from build123d import *

# Parameters (mm, degrees)
BOSS_EXTRUDE1_DEPTH = 25.4


with BuildPart() as part:
    # Sketch1 → Boss-Extrude1 (new body)
    with BuildSketch(Plane(origin=(0, 0, 0), x_dir=(1, 0, 0), z_dir=(0, 1, 0))):
        with BuildLine():
            Line((-2.032, 11.247927631), (-1.27, 14.803927631))
            Line((-1.27, 14.803927631), (1.27, 14.803927631))
            Line((1.27, 14.803927631), (2.032, 11.247927631))
            ThreePointArc((2.032, 11.247927631), (8.082230509, 8.082230509), (11.247927631, 2.032))
            Line((11.247927631, 2.032), (14.803927631, 1.27))
            Line((14.803927631, 1.27), (14.803927631, -1.27))
            Line((14.803927631, -1.27), (11.247927631, -2.032))
            ThreePointArc((11.247927631, -2.032), (8.082230509, -8.082230509), (2.032, -11.247927631))
            Line((2.032, -11.247927631), (1.27, -14.803927631))
            Line((1.27, -14.803927631), (-1.27, -14.803927631))
            Line((-1.27, -14.803927631), (-2.032, -11.247927631))
            ThreePointArc((-2.032, -11.247927631), (-8.082230509, -8.082230509), (-11.247927631, -2.032))
            Line((-11.247927631, -2.032), (-14.803927631, -1.27))
            Line((-14.803927631, -1.27), (-14.803927631, 1.27))
            Line((-14.803927631, 1.27), (-11.247927631, 2.032))
            ThreePointArc((-11.247927631, 2.032), (-8.082230509, 8.082230509), (-2.032, 11.247927631))
        make_face()
        with BuildLine():
            Line((-2.032, -1.524), (2.032, -1.524))
            ThreePointArc((2.032, -1.524), (0, 2.54), (-2.032, -1.524))
        make_face(mode=Mode.SUBTRACT)
    extrude(amount=BOSS_EXTRUDE1_DEPTH)


solid = part.part
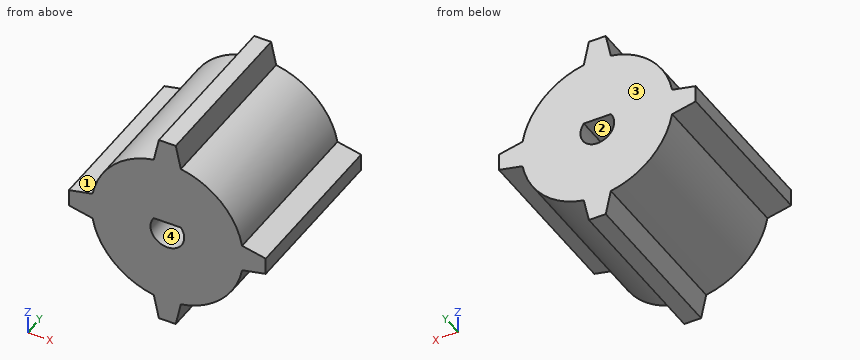
Model file for the job. Use its own axes, mm. Face numbers are marked on the shaded views. Round coordinates to 2 decimals unless told otherwise and drop trailing zeros. Order: outer loops, then holes, each group sorted by start corner. A loop starts at its lowest first (then second) coordinate and runs counter-clockwise, first axis right, second up. Notation, with made-up numbers: M 70,0.5 L 82,0.5 A28 cw 82,33.5 Z; hole C 49,-26.5 d11. An arc over 180 degrees is marked long. Write each question's results on one line, items separated by ' | '. Start each with the question number.
(1) Two-plate mould, pull along X, no slides. Class the marked faces 1, 2, 3 and 4: pulls with the +X half, pulls with the -X half, needs draft (parallel to the pull), parting line crosses it, or undercut.
(2) Saw through at B-B, the plane y = 13.75. Give the cut face in (x, z), then the cut area to 3 significant figures.
(3) Saw through at D-D, the plane x = 4.5. Give the cut face in (y, z), then the cut area to 3 significant figures.
(4) Probe probe 1 along X at (y, z) = (6, 0); probe 2 along X at (y, z) = (12.25, -2.25); probe 3 along Z at (x, y) = (-3.25, 2). List the from-to ranges inside material, lowest first. Write a range as from..to.
(5) Drop flat-ended pins along their axis: pin 1 (1 mm diameter, centred on x = 7.5, y = 6.5, fed in from +Z); pin 2 (4 mm diameter, centred on x = -11, y = 8.5, fed in from +Z); pin 3 (10 mm diameter, centred on y = 16, z = -5.5, fed in from -X); pin 4 (12 mm diameter, centred on y = 4.5, z = 11.5, fed in from +X). Give the stop position or say it passes through.
(6) Saw through at C-C, the plane x = 0. Give the cut face in (y, z).
(7) Saw through at A-A, the plane z = 0. Give the cut face in (x, y), then the cut area to 3 significant figures.
Established:
1) face 1: pulls with the -X half | face 2: undercut | face 3: needs draft | face 4: undercut
2) outline: M -14.8,-1.27 L -11.25,-2.03 A11.43 ccw -2.03,-11.25 L -1.27,-14.8 L 1.27,-14.8 L 2.03,-11.25 A11.43 ccw 11.25,-2.03 L 14.8,-1.27 L 14.8,1.27 L 11.25,2.03 A11.43 ccw 2.03,11.25 L 1.27,14.8 L -1.27,14.8 L -2.03,11.25 A11.43 ccw -11.25,2.03 L -14.8,1.27 Z; hole M -2.03,1.52 A2.54 ccw long 2.03,1.52 Z | area: 438 mm^2
3) outline: M 0,-10.51 L 25.4,-10.51 L 25.4,10.51 L 0,10.51 Z | area: 534 mm^2
4) probe 1: x = -14.8..-2.54, 2.54..14.8 | probe 2: x = -11.21..-1.18, 1.18..11.21 | probe 3: z = -10.96..10.96
5) pin 1: stops at z = 9.04 | pin 2: stops at z = 7.05 | pin 3: stops at x = -14.8 | pin 4: stops at x = 10.02
6) outline: M 0,-14.8 L 25.4,-14.8 L 25.4,-2.54 L 0,-2.54 Z; M 0,1.52 L 25.4,1.52 L 25.4,14.8 L 0,14.8 Z
7) outline: M -14.8,0 L -2.54,0 L -2.54,25.4 L -14.8,25.4 Z; M 2.54,0 L 14.8,0 L 14.8,25.4 L 2.54,25.4 Z | area: 623 mm^2
